The listing builds one solid part. Answer for the finished solid, in the listing's coordinates (mm). A direction names the side the tool comes from. Give positions to 0.01 mm unless a question says otherwise; leave off trailing zeros. Order: outer loops, then holes, each group sorted by start corner. A loop starts at its lowest first (then second) coordinate and runs counter-clockwise, first axis right, second up. Notation, with made-up numbers: (-4, 12.5) - (2, 12.5) arc R22 cw to (2, 38.5) - close; hole circle Ø6 at (-21, -10.5). An arc over 180 degrees is marked (long way). Write each question's results on one line, items separated by ' | '. Start each with the question number.
1. A flat-ended cylindrical pin translates along its axis: pin 1 (3 mm diameter, centred on y = 11, z = -0.5, fed in from +X). Find the tip coordinate at first contact, or state that the pin passes through.
2. Section B-B (x = 0) is taken. Give the vertices of the cut face in (y, z).
3. Find the intervals of material crossed by L1, parallel to Z at x = 0, y = 18.2; L2, parallel to Y at x = -1.25, z = -2.05; L3, parallel to Y at x = -0.25, z = 0.6, in increasing order.
4. Section A-A (y = 7.25) is taken. Give the vertices of the cut face in (x, z).
5. Which of the six approach directions +Z, -Z, +X, -X, +Y, -Y give full straight-line access (tool end or side, diameter ignored) to faces 1 (the face through (1, 20, -2)), 2 (the face through (0, 15, 0)), 3 (the face through (0.06, -2.71, -1.45))?
from build123d import *

# Parameters (mm, degrees)
BOSS_EXTRUDE1_DEPTH            = 20
SKETCH2_W                      = 1.45
SKETCH2_H                      = 6
F_2_9_2_9_DIAMETER_HOLE1_D     = 2.9
F_2_9_2_9_DIAMETER_HOLE1_DEPTH = 5
CHAMFER1_SIZE                  = 0.5


with BuildPart() as part:
    # Sketch1 → Boss-Extrude1 (new body)
    with BuildSketch(Plane(origin=(0, 20, 0), x_dir=(1, 0, 0), z_dir=(0, 1, 0))):
        Polygon((1.622354256, -2.81), (3.244708513, 0), (1.622354256, 2.81), (-1.622354256, 2.81), (-3.244708513, 0), (-1.622354256, -2.81), align=None)
    extrude(amount=-BOSS_EXTRUDE1_DEPTH)

    # Sketch2 → Revolve1 (revolve)
    with BuildSketch(Plane(origin=(0, 0, 0), x_dir=(-1, 0, 0), z_dir=(0, 0, -1)), mode=Mode.PRIVATE) as revolve1_sk:
        with Locations((-0.725, -3)):
            Rectangle(SKETCH2_W, SKETCH2_H)
    revolve(revolve1_sk.sketch.rotate(Axis((0, -6, 0), (0, 1, 0)), 270), axis=Axis((0, -6, 0), (0, 1, 0)))

    # Ø2.9 (2.9) Diameter Hole1
    with Locations(Plane(origin=(0, 20, 0), x_dir=(1, 0, 0), z_dir=(0, 1, 0))):
        with Locations((0, 0)):
            Hole(F_2_9_2_9_DIAMETER_HOLE1_D / 2, depth=F_2_9_2_9_DIAMETER_HOLE1_DEPTH)

    # Chamfer1
    chamfer1_edges = [part.edges().sort_by_distance(p)[0] for p in [
        (0, -6, -1.45),
        (1.45, 20, 0),
    ]]
    chamfer(chamfer1_edges, length=CHAMFER1_SIZE)


solid = part.part
Reported:
1) pin 1: x = 3.24
2) outline: (-6, -0.95) - (-5.5, -1.45) - (0, -1.45) - (0, -2.81) - (20, -2.81) - (20, -1.95) - (19.5, -1.45) - (15, -1.45) - (15, 1.45) - (19.5, 1.45) - (20, 1.95) - (20, 2.81) - (0, 2.81) - (0, 1.45) - (-5.5, 1.45) - (-6, 0.95) - close
3) L1: -2.81 to -1.45, 1.45 to 2.81 | L2: 0 to 20 | L3: -6 to 15
4) outline: (-3.24, 0) - (-1.62, -2.81) - (1.62, -2.81) - (3.24, 0) - (1.62, 2.81) - (-1.62, 2.81) - close
5) face 1: +Z, -Z, +X, -X, +Y | face 2: +Y | face 3: -Y
